Verification items for the finished model (mm, model axes). A direction names the side the tool comes from. Coordinates: 2 decimals unless noted, no trailing zeros. Order: outer loops, then holes, each group sorted by start corner. A loop starts at its lowest first (then second) coordinate and runs counter-clockwise, first axis right, second up. Notation, with made-up numbers: M -28.5,6.5 L 4.5,6.5 A12 ccw 4.5,11.5 Z; hole C 81,-21 d8. An arc over 180 degrees is marked long. Write item = value, one per line.
```python
from build123d import *

# Parameters (mm, degrees)
F0_R     = 5
F0_R_2   = 2
F1_DEPTH = 1
F2_R     = 3
F2_R_2   = 2
F3_DEPTH = 1
F4_W     = 2.446195
F4_H     = 0.930616
F5_DEPTH = 1
F6_R     = 0.2


with BuildPart() as f1:
    # F0 (on Top) → F1 (new body)
    with BuildSketch(Plane.XY):
        Circle(F0_R)
        Circle(F0_R_2, mode=Mode.SUBTRACT)
    extrude(amount=F1_DEPTH)

    # F2 (on face) → F3 (join)
    with BuildSketch(Plane.XY.offset(1)):
        Circle(F2_R)
        Circle(F2_R_2, mode=Mode.SUBTRACT)
    extrude(amount=F3_DEPTH)

    # F4 (on face) → F5 (cut)
    with BuildSketch(Plane.XY.offset(2)):
        with Locations((2.446193, 0)):
            Rectangle(F4_W, F4_H)
    extrude(amount=-F5_DEPTH, mode=Mode.SUBTRACT)

    # F6
    f6_edges = [f1.edges().sort_by_distance(p)[0] for p in [
        (-5, 0, 1),
    ]]
    fillet(f6_edges, radius=F6_R)


solid = f1.part
```
Item 1: Scan lines: L1, parallel to Y at x = -4, z = 0.6; L2, parallel to Z at x = -2, y = -3.25; L3, parallel to Y at x = 0.75, z = 1.4. Record each from-to range of solid material in increasing order. Write a range as from..to.
Report:
L1 = -3..3
L2 = 0..1
L3 = -2.9..-1.85, 1.85..2.9
Item 2: Release check for a two-part mould opening along Y. For faces 1 (the flat face through (2, -1, 2)), 2 (the cylindrical face through (-1.08, -4.88, 0.39)), 3 (the flat face through (2.4, -0.465, 1.5)) record: pulls with the +Y half, pulls with the -Y half, needs draft (parallel to the pull), parting line crosses it, or undercut.
Report:
face_1 = needs draft
face_2 = parting line crosses it
face_3 = undercut
Item 3: Tool access check on faces 4 (the flat face through (-0.1, -2.2, 0)), 5 (the cylindrical face through (-3, 0.1, 1.5)), 6 (the flat face through (2.4, 0.465, 1.5)). Record the directions out of +Z, -Z, +X, -X, +Y, -Y that give a thin tool (end or side, any length) a straight path to the whole face; none if there is none.
Report:
face_4 = -Z, +X, -X, +Y, -Y
face_5 = +Z
face_6 = +Z, +X
Item 4: Sectioned sample at A-A, the plane x = 0. Enter the section's corners in (y, z), then the cut area to 3 significant figures.
Report:
outline = M -5,0 L -2,0 L -2,2 L -3,2 L -3,1 L -4.8,1 A0.2 ccw -5,0.8 Z; M 2,0 L 5,0 L 5,0.8 A0.2 ccw 4.8,1 L 3,1 L 3,2 L 2,2 Z
area = 7.98 mm^2
Item 5: Sectioned sample at C-C, the plane z = 1.6. Enter the section's corners in (x, y).
Report:
outline = M 1.95,-0.47 A2 cw long 1.95,0.47 L 2.96,0.47 A3 ccw long 2.96,-0.47 Z
Item 6: Gauge pin test, flat ends, axial feed: pin 1 (0.5 mm diameter, centred on x = 2.5, z = 1.5, fed in from -Y); pin 2 (0.8 mm diameter, centred on x = 2, z = 1.5, fed in from +Y). Record the tip position at first contact, or that the pin passes through.
Report:
pin_1 = -1.98
pin_2 = 2.54
Item 7: Sectioned sample at B-B, the plane y = 0. Enter the section's corners in (x, z), then the cut area to 3 significant figures.
Report:
outline = M -5,0 L -2,0 L -2,2 L -3,2 L -3,1 L -4.8,1 A0.2 ccw -5,0.8 Z; M 2,0 L 5,0 L 5,0.8 A0.2 ccw 4.8,1 L 2,1 Z
area = 6.98 mm^2
